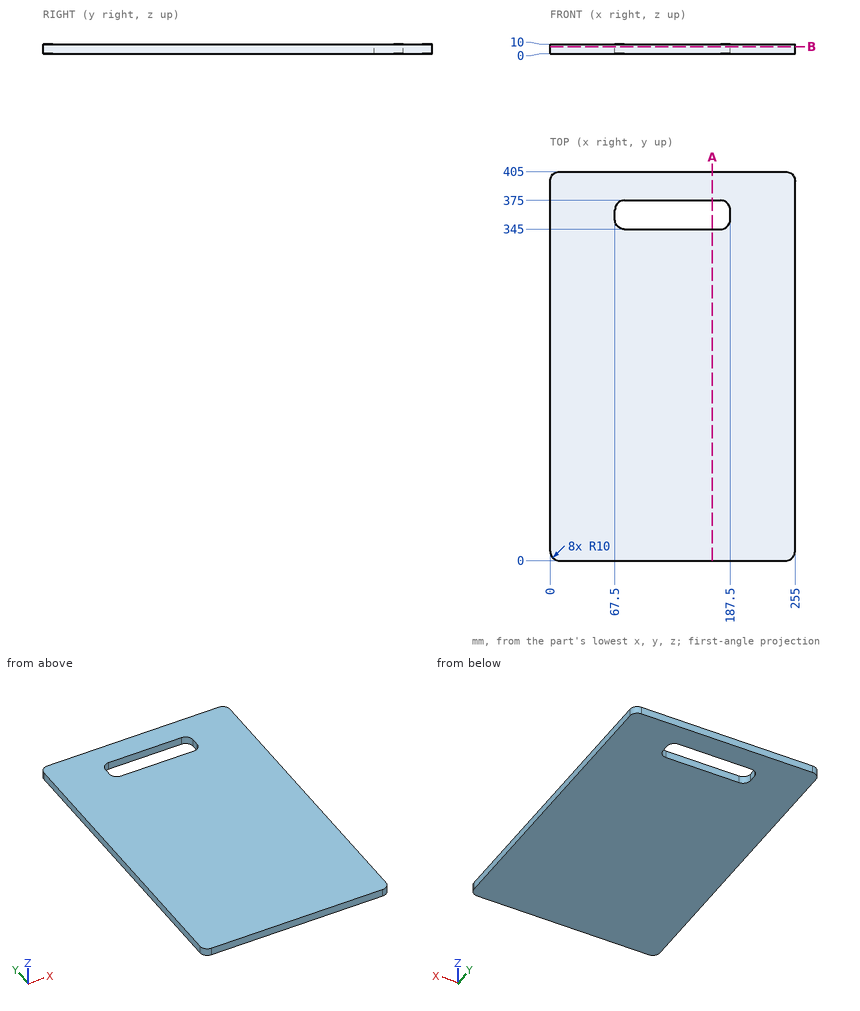
For this review, use the dimensioned drawing (mm, ordinates from the lowest corner) and the shaded views. Coordinates: 2 decimals unless noted, no trailing zeros. Loops run counter-clockwise (first coordinate to the right, second up) from the corner with the lowest first, then second, coordinate; pieces in that order, holes last. Notation, with made-up numbers: (-10, 46) -> (38, 46) arc R25 cw to (38, 67) -> close; hole circle Ø8 at (27, -32.5). An arc over 180 degrees is marked (long way). Use a Markdown table: item, result. Add a question column.
1. To check wall thickness, follow line 1 (Y direction, x = 96.5, z = 8.25); line 2 (Y direction, x = 69, z = 0.75); line 3 (X direction, y = 369, z = 1.75). State the ranges of each line that lie inside material, in increasing order.
2. Add section A-A on x = 169. Write out the cut boundary in (y, z).
3. Add section B-B on z = 7.25. Write out the cut boundary in (x, y).
Returned:
| question | item | result |
|---|---|---|
| 1 | line 1 | y = 0 to 345, 375 to 405 |
| 1 | line 2 | y = 0 to 349.73, 370.27 to 405 |
| 1 | line 3 | x = 0 to 68.33, 186.67 to 255 |
| 2 | outline | (0, 0) -> (345, 0) -> (345, 10) -> (0, 10) -> close; (375, 0) -> (405, 0) -> (405, 10) -> (375, 10) -> close |
| 3 | outline | (0, 10) arc R10 ccw to (10, 0) -> (245, 0) arc R10 ccw to (255, 10) -> (255, 395) arc R10 ccw to (245, 405) -> (10, 405) arc R10 ccw to (0, 395) -> close; hole (67.5, 355) arc R10 ccw to (77.5, 345) -> (177.5, 345) arc R10 ccw to (187.5, 355) -> (187.5, 365) arc R10 ccw to (177.5, 375) -> (77.5, 375) arc R10 ccw to (67.5, 365) -> close |
